Here's how the part is built. I have some questions about the finished solid (model axes, mm). A direction names the side the tool comes from. Coordinates: 2 decimals unless noted, no trailing zeros. Loops run counter-clockwise (first coordinate to the right, second up) from the corner with the lowest first, then second, coordinate; pieces in that order, holes last. Notation, with made-up numbers: (-30, -29.75) - (12, -29.75) arc R8 ccw to (12, -15.75) - close; hole circle Ø11 at (56, 5). An arc over 180 degrees is marked (long way). Use a Markdown table: item, result.
```python
from build123d import *

# Parameters (mm, degrees)
F0_W     = 25.4
F0_H     = 25.4
F1_DEPTH = 750
F2_T     = -2
F3_R     = 4.5
F4_DEPTH = 1.6
F5_R     = 4.5
F6_DEPTH = 1.6


with BuildPart() as f1:
    # F0 (on Right) → F1 (new body, symmetric)
    with BuildSketch(Plane.YZ):
        Rectangle(F0_W, F0_H)
    extrude(amount=F1_DEPTH, both=True)

    # F2
    f2_openings = [f1.faces().sort_by_distance(p)[0] for p in [
        (750, 0, 0),
        (-750, 0, 0),
    ]]
    offset(amount=F2_T, openings=f2_openings)

    # F3 (on face) → F4 (join)
    with BuildSketch(Plane.YZ.offset(750)):
        with BuildLine():
            ThreePointArc((42.7, 10.7), (42.114214, 12.114214), (40.7, 12.7))
            Line((40.7, 12.7), (-40.7, 12.7))
            ThreePointArc((-40.7, 12.7), (-42.114214, 12.114214), (-42.7, 10.7))
            Line((-42.7, 10.7), (-42.7, -10.7))
            ThreePointArc((-42.7, -10.7), (-42.114214, -12.114214), (-40.7, -12.7))
            Line((-40.7, -12.7), (40.7, -12.7))
            ThreePointArc((40.7, -12.7), (42.114214, -12.114214), (42.7, -10.7))
            Line((42.7, -10.7), (42.7, 10.7))
        make_face()
        with Locations((-27.7, 0)):
            Circle(F3_R, mode=Mode.SUBTRACT)
        with Locations((27.7, 0)):
            Circle(F3_R, mode=Mode.SUBTRACT)
    extrude(amount=F4_DEPTH)

    # F5 (on face) → F6 (join)
    with BuildSketch(Plane(origin=(-750, 0, 0), x_dir=(0, -1, 0), z_dir=(-1, 0, 0))):
        with BuildLine():
            Line((-12.7, 12.7), (-40.7, 12.7))
            ThreePointArc((-40.7, 12.7), (-42.114214, 12.114214), (-42.7, 10.7))
            Line((-42.7, 10.7), (-42.7, -10.7))
            ThreePointArc((-42.7, -10.7), (-42.114214, -12.114214), (-40.7, -12.7))
            Line((-40.7, -12.7), (-12.7, -12.7))
            Line((-12.7, -12.7), (-12.7, 12.7))
        make_face()
        with Locations((-27.7, 0)):
            Circle(F5_R, mode=Mode.SUBTRACT)
        with BuildLine():
            Line((12.7, 12.7), (-12.7, 12.7))
            Line((-12.7, 12.7), (-12.7, -12.7))
            Line((-12.7, -12.7), (12.7, -12.7))
            Line((12.7, -12.7), (40.7, -12.7))
            ThreePointArc((40.7, -12.7), (42.114214, -12.114214), (42.7, -10.7))
            Line((42.7, -10.7), (42.7, 10.7))
            ThreePointArc((42.7, 10.7), (42.114214, 12.114214), (40.7, 12.7))
            Line((40.7, 12.7), (12.7, 12.7))
        make_face()
        with Locations((27.7, 0)):
            Circle(F5_R, mode=Mode.SUBTRACT)
    extrude(amount=F6_DEPTH)


solid = f1.part
```
Q1. If we mould it in two halves opening along X, with no side actions, what happens to faces 1 (the face through (750, 24, 3)), 2 (the face through (4, 6, -12.7)), 3 (the face through (751.6, -1, 0)), 4 (the face through (10, 12.7, 0))? For each: pulls with the +X half, pulls with the -X half, needs draft (parallel to the pull), parting line crosses it, or undercut.
Check values:
| item | result |
|---|---|
| face 1 | undercut |
| face 2 | needs draft |
| face 3 | pulls with the +X half |
| face 4 | undercut |
Q2. I want a section at A-A, the plane x = -72. Write out the boundary of the cut face in (y, z).
Check values:
| item | result |
|---|---|
| outline | (-12.7, -12.7) - (12.7, -12.7) - (12.7, 12.7) - (-12.7, 12.7) - close; hole (-10.7, -10.7) - (10.7, -10.7) - (10.7, 10.7) - (-10.7, 10.7) - close |
Q3. Will this pin go through, and if not, where does the flat tip stop? P1, Ø1.5, axis at x = 197, z = 5, coming from the +Y side.
Check values:
| item | result |
|---|---|
| P1 | y = 12.7 |
Q4. Which directions (+Z, -Z, +X, -X, +Y, -Y) give clear straight access to the entire face, cutting with the end or side of a thin tool? Please do faces 5 (the face through (-751.6, 1, 0)), 6 (the face through (-750, -24, 3)), 7 (the face through (-750, 28, 6)).
Check values:
| item | result |
|---|---|
| face 5 | +Z, -Z, -X, +Y, -Y |
| face 6 | +Z, -Z, -Y |
| face 7 | +Z, -Z, +Y |
Q5. Please list where these lines run through material, in increasing order: L1, parallel to X at y = -28.5, z = 7; L2, parallel to Z at x = -751, y = 27; L3, parallel to Y at x = 572, z = 6.75. Write a range as from..to.
Check values:
| item | result |
|---|---|
| L1 | -751.6..-750, 750..751.6 |
| L2 | -12.7..-4.45, 4.45..12.7 |
| L3 | -12.7..-10.7, 10.7..12.7 |
Q6. I want a section at B-B, the plane z = 0. Give the number of separate pieces and of enclosed holes in the cut face, then the cut area to 3 significant figures.
Check values:
| item | result |
|---|---|
| separate pieces | 5 |
| enclosed holes | 1 |
| area | 6,220 mm^2 |
